Input: part model. Units: mm. Frame: model coordinates. A direction names the side the tool comes from. Give positions to 0.01 mm unless a question says otherwise; leave off trailing zeros. Loops run counter-clockwise (first coordinate to the right, second up) from the corner with the lowest first, then second, coordinate; pieces in that order, holes last. Notation, with made-up numbers: (-35, 16) -> (2, 16) arc R9 ccw to (2, 22) -> close; hole circle Ø6 at (70, 58.5). An arc over 180 degrees is marked (long way). Answer as a JSON object with one key per item and string values.
```python
from build123d import *

# Parameters (mm, degrees)
F0_R     = 0.85
F1_DEPTH = 1


with BuildPart() as f1:
    # F0 (on Top) → F1 (new body)
    with BuildSketch(Plane.XY):
        with BuildLine():
            ThreePointArc((-0.25, -7.595887), (0, 7.6), (0.25, -7.595887))
            Line((0.25, -7.595887), (0.25, -11.297234))
            ThreePointArc((0.25, -11.297234), (1.431103, -11.209012), (2.596485, -10.997648))
            ThreePointArc((2.596485, -10.997648), (3.006169, -10.755478), (3.205819, -10.323475))
            Line((3.205819, -10.323475), (3.328522, -9.391454))
            ThreePointArc((3.328522, -9.391454), (3.747523, -8.281762), (4.615831, -7.473667))
            ThreePointArc((4.615831, -7.473667), (0, 9.9), (-4.615831, -7.473667))
            ThreePointArc((-4.615831, -7.473667), (-3.747523, -8.281762), (-3.328522, -9.391454))
            Line((-3.328522, -9.391454), (-3.205819, -10.323475))
            ThreePointArc((-3.205819, -10.323475), (-3.006169, -10.755478), (-2.596485, -10.997648))
            ThreePointArc((-2.596485, -10.997648), (-1.431103, -11.209012), (-0.25, -11.297234))
            Line((-0.25, -11.297234), (-0.25, -7.595887))
        make_face()
        with Locations((-1.35, -9.6)):
            Circle(F0_R, mode=Mode.SUBTRACT)
        with Locations((1.35, -9.6)):
            Circle(F0_R, mode=Mode.SUBTRACT)
    extrude(amount=F1_DEPTH)


solid = f1.part
```
Q1. Section B-B, the plane x = 1.35. Return the cut outline in (y, z).
Evaluation:
{"outline": "(-11.22, 0) -> (-10.45, 0) -> (-10.45, 1) -> (-11.22, 1) -> close; (-8.75, 0) -> (-7.48, 0) -> (-7.48, 1) -> (-8.75, 1) -> close; (7.48, 0) -> (9.8, 0) -> (9.8, 1) -> (7.48, 1) -> close"}
Q2. Section D-D, the plane x = 4.25. Return the cut outline in (y, z).
Evaluation:
{"outline": "(-7.73, 0) -> (-6.3, 0) -> (-6.3, 1) -> (-7.73, 1) -> close; (6.3, 0) -> (8.87, 0) -> (8.87, 1) -> (6.3, 1) -> close"}
Q3. Section A-A, the plane z = 0.4. Return the cut outline in (x, y), then the cut area to 3 significant figures.
Evaluation:
{"outline": "(-4.62, -7.47) arc R2.6 cw to (-3.33, -9.39) -> (-3.21, -10.32) arc R0.8 ccw to (-2.6, -11) arc R11.3 ccw to (-0.25, -11.3) -> (-0.25, -7.6) arc R7.6 cw (long way) to (0.25, -7.6) -> (0.25, -11.3) arc R11.3 ccw to (2.6, -11) arc R0.8 ccw to (3.21, -10.32) -> (3.33, -9.39) arc R2.6 cw to (4.62, -7.47) arc R9.3 ccw (long way) to start; hole circle Ø1.7 at (-1.35, -9.6); hole circle Ø1.7 at (1.35, -9.6)", "area": "102 mm2"}
Q4. Access query for faces 1 (the cylindrical face through (0.5, -9.6, 0.5)), 2 (the flat face through (-0.25, -9.5, 0.5)). Directions: +Z, -Z, +X, -X, +Y, -Y. A direction counts if a zero-diameter tool reaches every point of the face in a straight line with its end or side. Return the directions, or none.
Evaluation:
{"face 1": "+Z, -Z", "face 2": "+Z, -Z, -Y"}
Q5. Pin query (flat end, axial travel): pin 1 (3 mm diameter, centred on x = -4, y = -4.5, fed in from +Z). Return the tip coordinate at first contact, or that it passes through.
Evaluation:
{"pin 1": "passes through"}
Q6. Section C-C, the plane y = 0.6. Return the cut outline in (x, z), then the cut area to 3 significant figures.
Evaluation:
{"outline": "(-9.3, 0) -> (-7.58, 0) -> (-7.58, 1) -> (-9.3, 1) -> close; (7.58, 0) -> (9.3, 0) -> (9.3, 1) -> (7.58, 1) -> close", "area": "3.45 mm2"}
Q7. Ray query, line 1 along Y through (x, z) = (-1.35, 0.35); line 2 along Y through (x, z) = (2, 0.2); line 3 along X through (y, z) = (-6, 0.1). Return the intervals inside material, ascending.
Evaluation:
{"line 1": "y = -11.22 to -10.45, -8.75 to -7.48, 7.48 to 9.8", "line 2": "y = -11.12 to -10.15, -9.05 to -7.33, 7.33 to 9.68", "line 3": "x = -6.55 to -4.66, 4.66 to 6.55"}
Q8. Draft query along X for faces 3 (the flat face through (0.25, -9.4, 0.5)), 4 (the flat face through (-3.5, 7.2, 1)), 5 (the flat face through (3.266, -9.864, 0.493)). Return one class per face: +X half, -X half, draft (parallel to the pull), parting line (faces both ways), or undercut.
Evaluation:
{"face 3": "undercut", "face 4": "draft", "face 5": "+X half"}
